The model under review builds one solid part; all positions refer to its coordinate system, in mm. A direction names the side the tool comes from. Coordinates: 2 decimals unless noted, no trailing zeros. Order: outer loops, then holes, each group sorted by start corner. A loop starts at its lowest first (then second) coordinate and runs counter-clockwise, first axis right, second up. Notation, with made-up numbers: (-38.5, 81) -> (-30.5, 81) arc R16 cw to (-30.5, 100) -> close; hole circle Ø4 at (-22, 7.25). An arc over 180 degrees is marked (long way). Use CSV: the item, a comma, the result in double quotes. Start each with the question number.
```python
from build123d import *

# Parameters (mm, degrees)
EXTRUDE_1_DEPTH          = 30
CUT_EXTRUDE_1_DEPTH      = 30
CUT_EXTRUDE_1_DEPTH_BACK = 30
SKETCH_2_W               = 4.827470223
SKETCH_2_H               = 5.659354242
FILLET_1_R               = 11
SKETCH_3_R               = 1.5
CUT_EXTRUDE_2_DEPTH      = 30
SKETCH_4_R               = 1
SKETCH_4_R_2             = 1.25
CUT_EXTRUDE_3_DEPTH      = 43.640942766
FILLET_2_R               = 1
FILLET_3_R               = 0.2
FILLET_4_R               = 2
FILLET_5_R               = 2


# Some blends are built 0.0001 mm under size
with BuildPart() as part:
    # 草图1 → 凸台-拉伸1 (new body)
    with BuildSketch(Plane.XY):
        Polygon((0, 0), (18.5, 0), (20, 0), (20, 24), (18.5, 24), (18.5, 1.5), (0, 1.5), align=None)
    extrude(amount=EXTRUDE_1_DEPTH)

    # 草图2 → 切除-拉伸1 (cut, two sides: drawn at the far end of the back side and taken through both)
    with BuildSketch(Plane(origin=(0, 1.5, 0), x_dir=(1, 0, 0), z_dir=(0, 1, 0)).offset(-CUT_EXTRUDE_1_DEPTH_BACK)):
        with Locations((19.913735112, -1.170322879)):
            Rectangle(SKETCH_2_W, SKETCH_2_H)
        with Locations((19.913735112, -28.829677121)):
            Rectangle(SKETCH_2_W, SKETCH_2_H)
    extrude(amount=CUT_EXTRUDE_1_DEPTH + CUT_EXTRUDE_1_DEPTH_BACK, mode=Mode.SUBTRACT)

    # 圆角1
    fillet_1_edges = [part.edges().sort_by_distance(p)[0] for p in [
        (19.25, 24, 26),
        (19.25, 24, 4),
    ]]
    fillet(fillet_1_edges, radius=FILLET_1_R - 0.0001)  # a hair under: the kernel refuses the full size

    # 草图3 → 切除-拉伸2 (cut)
    with BuildSketch(Plane(origin=(0, 1.5, 0), x_dir=(1, 0, 0), z_dir=(0, 1, 0))):
        with Locations(Location((13.5, -4, 0), (0, 0, 270))):
            Circle(SKETCH_3_R)
        with Locations(Location((3.5, -4, 0), (0, 0, 270))):
            Circle(SKETCH_3_R)
        with Locations(Location((3.5, -26, 0), (0, 0, 270))):
            Circle(SKETCH_3_R)
        with Locations(Location((13.5, -26, 0), (0, 0, 270))):
            Circle(SKETCH_3_R)
        with BuildLine():
            Line((7.5, -9), (11.5, -9))
            ThreePointArc((11.5, -9), (12.914213562, -9.585786438), (13.5, -11))
            Line((13.5, -11), (13.5, -19))
            ThreePointArc((13.5, -19), (12.914213562, -20.414213562), (11.5, -21))
            Line((11.5, -21), (7.5, -21))
            ThreePointArc((7.5, -21), (6.085786438, -20.414213562), (5.5, -19))
            Line((5.5, -19), (5.5, -11))
            ThreePointArc((5.5, -11), (6.085786438, -9.585786438), (7.5, -9))
        make_face()
    extrude(amount=-CUT_EXTRUDE_2_DEPTH, mode=Mode.SUBTRACT)

    # 草图4 → 切除-拉伸3 (cut, through all)
    with BuildSketch(Plane.ZY.offset(-18.5)):
        with Locations((8, 13)):
            Circle(SKETCH_4_R)
        with Locations(Location((22, 13, 0), (0, 0, 180))):
            Circle(SKETCH_4_R)
        with Locations((9, 10)):
            Circle(SKETCH_4_R_2)
        with Locations(Location((21, 10, 0), (0, 0, 180))):
            Circle(SKETCH_4_R_2)
        with BuildLine():
            Line((16, 8.101020514), (16, 4.101020514))
            Line((16, 4.101020514), (14, 4.101020514))
            Line((14, 4.101020514), (14, 8.101020514))
            ThreePointArc((14, 8.101020514), (10, 13), (14, 17.898979486))
            Line((14, 17.898979486), (14, 21.898979486))
            Line((14, 21.898979486), (16, 21.898979486))
            Line((16, 21.898979486), (16, 17.898979486))
            ThreePointArc((16, 17.898979486), (20, 13), (16, 8.101020514))
        make_face()
    extrude(amount=-CUT_EXTRUDE_3_DEPTH, mode=Mode.SUBTRACT)

    # 圆角2
    fillet_2_edges = [part.edges().sort_by_distance(p)[0] for p in [
        (19.25, 4.101020514, 14),
        (19.25, 4.101020514, 16),
        (19.25, 21.898979486, 16),
        (19.25, 21.898979486, 14),
    ]]
    fillet(fillet_2_edges, radius=FILLET_2_R - 0.0001)  # a hair under: the kernel refuses the full size

    # 圆角3
    fillet_3_edges = [part.edges().sort_by_distance(p)[0] for p in [
        (19.25, 8.101020514, 14),
        (19.25, 17.898979486, 14),
        (19.25, 17.898979486, 16),
        (19.25, 8.101020514, 16),
    ]]
    fillet(fillet_3_edges, radius=FILLET_3_R)

    # 圆角4
    # the kernel refuses this fillet: 2 mm, written as the material it adds along each edge
    with BuildSketch(Plane(origin=(17.5, 0, 26), x_dir=(1, 0, 0), z_dir=(0, 1, 0))) as fillet_4_piece_1:
        with BuildLine():
            CenterArc((FILLET_4_R, -FILLET_4_R), FILLET_4_R, 90, 90)
            Line((0, -FILLET_4_R), (0, 0))
            Line((0, 0), (FILLET_4_R, 0))
        make_face()
    extrude(amount=1.5)
    with BuildSketch(Plane(origin=(17.5, 0, 4), x_dir=(1, 0, 0), z_dir=(0, 1, 0))) as fillet_4_piece_2:
        with BuildLine():
            CenterArc((FILLET_4_R, FILLET_4_R), FILLET_4_R, 180, 90)
            Line((0, FILLET_4_R), (0, 0))
            Line((0, 0), (FILLET_4_R, 0))
        make_face()
    extrude(amount=1.5)
    # the kernel refuses this fillet: 2 mm, written as the material it takes off along each edge
    with BuildSketch(Plane(origin=(17.5, 6.5, 0), x_dir=(0, 0, 1), z_dir=(0, -1, 0)), Plane(origin=(17.5, -5, 30), x_dir=(0, 0, -1), z_dir=(0, 1, 0)), Plane(origin=(0, 6.5, 30), x_dir=(0, 0, -1), z_dir=(0, -1, 0)), Plane(origin=(0, 6.5, 0), x_dir=(1, 0, 0), z_dir=(0, -1, 0))) as fillet_4_2_piece_1:
        with BuildLine():
            CenterArc((FILLET_4_R, FILLET_4_R), FILLET_4_R, 180, 90)
            Line((0, FILLET_4_R), (0, 0))
            Line((0, 0), (FILLET_4_R, 0))
        make_face()
    extrude(amount=11.5, mode=Mode.SUBTRACT)

    # 圆角5
    fillet_5_edges = [part.edges().sort_by_distance(p)[0] for p in [
        (20, 0, 15),
        (18.5, 1.5, 15),
    ]]
    fillet(fillet_5_edges, radius=FILLET_5_R)


solid = part.part
```
Q1. Draft analysis for pull direction X (two halves, no side actions). For faces 1 (the cylindrical face through (19.26, 21.598, 15.715)), 2 (the flat face through (9, 1, 9)), 3 (the cylindrical face through (12.93, 0.76, 20.4)), 4 (the flat face through (20, 8, 17)), state which applies: +X half, -X half, draft (parallel to the pull), parting line (faces both ways), or undercut.
Q2. Add section B-B, the plane z = 25. State the section outline as (x, y) points, then the cut area to 3 significant figures.
Q3. To check wall thickness, follow probe 1 along Y at (x, z) = (19.1, 22); probe 2 along Y at (x, z) = (19.5, 22); probe 3 along Y at (x, z) = (15, 27.5). State the ranges of each line that lie inside material, in increasing order.
Q4. Clearance check with flat-ended pins moving along their axes: pin 1 Ø5 at (y, z) = (20.5, 4) entering from -X; pin 2 Ø3 at (x, y) = (18.5, 4) entering from +Z; pin 3 Ø10 at (x, z) = (9.5, 25) entering from +Y. State where each tip first meets the part, or that it passes through.
Q5. Add section C-C, the plane y = 20. State the section outline as (x, z) points.
Q6. Add section A-A, the plane x = 11. State the section outline as (y, z) points, then the cut area to 3 significant figures.
Q7. For faces 5 (the cylindrical face through (0.57, 0.76, 0.6)), 6 (the flat face through (18.5, 11.6, 10)), 7 (the cylindrical face through (19.26, 4.386, 15.699)), list the 3-axis set-ups (+Z, -Z, +X, -X, +Y, -Y) from which the entire face can be reached by the end or side of a thin tool; tool diameter is ignored.
Q8. Add section D-D, the plane z = 6.25. State the section outline as (x, y) points, then the cut area to 3 significant figures.
Answer block:
1,face 1,"draft"
1,face 2,"undercut"
1,face 3,"undercut"
1,face 4,"+X half"
2,outline,"(0, 0) -> (2.38, 0) -> (2.38, 1.5) -> (0, 1.5) -> close; (4.62, 0) -> (12.38, 0) -> (12.38, 1.5) -> (4.62, 1.5) -> close; (14.62, 0) -> (18, 0) arc R2 ccw to (20, 2) -> (20, 17.58) -> (18.5, 17.58) -> (18.5, 3.5) arc R2 cw to (16.5, 1.5) -> (14.62, 1.5) -> close"
2,area,"47.4 mm²"
3,probe 1,"y = 0.33 to 9.25, 10.75 to 12, 14 to 21.49"
3,probe 2,"y = 0.68 to 9.25, 10.75 to 12, 14 to 21.49"
3,probe 3,"y = 0 to 1.5"
4,pin 1,"stops at x = 18.5"
4,pin 2,"stops at z = 26"
4,pin 3,"stops at y = 1.5"
5,outline,"(18.5, 6.51) -> (20, 6.51) -> (20, 14) -> (18.5, 14) -> close; (18.5, 16) -> (20, 16) -> (20, 23.49) -> (18.5, 23.49) -> close"
6,outline,"(0, 0) -> (1.5, 0) -> (1.5, 9) -> (0, 9) -> close; (0, 21) -> (1.5, 21) -> (1.5, 30) -> (0, 30) -> close"
6,area,"27.0 mm²"
7,face 5,"-Z, -X, +Y, -Y"
7,face 6,"+Z, -Z, -X, +Y"
7,face 7,"+X, -X"
8,outline,"(0, 0) -> (18, 0) arc R2 ccw to (20, 2) -> (20, 19.67) -> (18.5, 19.67) -> (18.5, 3.5) arc R2 cw to (16.5, 1.5) -> (0, 1.5) -> close"
8,area,"57.2 mm²"
